```python
from build123d import *

# Parameters (mm, degrees)
F0_W          = 30
F0_H          = 50
F1_DEPTH      = 10
F2_R          = 10.0991386475
F3_DEPTH      = 10
F4_R          = 4.0969126616
F5_DEPTH      = 25
F5_DEPTH_BACK = 25
F6_SIZE       = 0.5
F7_SIZE       = 0.5


# Not quite as in the source:
# - a feature names something its author has since deleted; it is built from what else it names


with BuildPart() as f1:
    # F0 (on Top) → F1 (new body)
    with BuildSketch(Plane.XY):
        Rectangle(F0_W, F0_H)
    extrude(amount=-F1_DEPTH)

    # F2 (on Top) → F3 (join)
    with BuildSketch(Plane.XY):
        Circle(F2_R)
    extrude(amount=F3_DEPTH)

    # F4 (on Top) → F5 (cut, two sides)
    with BuildSketch(Plane.XY) as f5_sk:
        Circle(F4_R)
    extrude(amount=-F5_DEPTH, mode=Mode.SUBTRACT)
    extrude(f5_sk.sketch, amount=F5_DEPTH_BACK, mode=Mode.SUBTRACT)

    # F6
    f6_edges = [f1.edges().sort_by_distance(p)[0] for p in [
        (15, 0, 0),
        (0, -25, 0),
        (-15, 0, 0),
        (0, 25, 0),
        (-10.099139, 0, 10),
        (-4.096913, 0, 10),
        (15, -25, -5),
        (15, 25, -5),
        (-15, -25, -5),
        (0, -25, -10),
        (15, 0, -10),
        (-15, 25, -5),
        (-15, 0, -10),
        (0, 25, -10),
    ]]
    chamfer(f6_edges, length=F6_SIZE)

    # F7
    f7_edges = [f1.edges().sort_by_distance(p)[0] for p in [
        (-4.096913, 0, -10),
    ]]
    chamfer(f7_edges, length=F7_SIZE)


solid = f1.part
```
The listing builds one solid part. Answer for the finished solid, in the listing's coordinates (mm). Give positions to 0.01 mm unless a question says otherwise; leave off trailing zeros. Order: outer loops, then holes, each group sorted by start corner. A loop starts at its lowest first (then second) coordinate and runs counter-clockwise, first axis right, second up.
Item 1: Find the intervals of material crossed by probe 1 along Y at (x, z) = (0, 0.5); probe 2 along X at (y, z) = (0, -3.5); probe 3 along Z at (x, y) = (-13, 23.5), in increasing order.
From the geometry:
probe 1: y = -10.1 to -4.1, 4.1 to 10.1
probe 2: x = -15 to -4.1, 4.1 to 15
probe 3: z = -10 to 0
Item 2: Given pin 1 Ø6 at (y, z) = (11, 7.5) entering from +X; pin 2 Ø1 at (x, y) = (0, -4) entering from -Z; pin 3 Ø5 at (x, y) = (-10, 12) entering from +Z; pin 4 Ø5 at (x, y) = (0, 0) entering from +Z, each flat-ended and moving along its own axis, determine where each tip first touches the part or whether it passes through.
From the geometry:
pin 1: stops at x = 6.16
pin 2: stops at z = -9.9
pin 3: stops at z = 0
pin 4: passes through
Item 3: For a pull along Y with two mould halves and no side action, classify faces 1 (the face through (0, 6, -10)), 2 (the face through (0, 25, -5)), 3 (the face through (9.633, 3.034, 4.684)), 4 (the face through (3.91, 1.23, 0.13)) as pulls with the +Y half, pulls with the -Y half, needs draft (parallel to the pull), parting line crosses it, or undercut.
From the geometry:
face 1: needs draft
face 2: pulls with the +Y half
face 3: parting line crosses it
face 4: undercut
Item 4: The part is cut by section D-D, the plane y = 14. Give the vertices of the cut face in (x, z).
From the geometry:
outline: (-15, -9.5) - (-14.5, -10) - (14.5, -10) - (15, -9.5) - (15, -0.5) - (14.5, 0) - (-14.5, 0) - (-15, -0.5) - close
Item 5: The part is cut by section C-C, the plane z = -5.25. Give the vertices of the cut face in (x, y), and give its area (3 significant figures).
From the geometry:
outline: (-15, -24.5) - (-14.5, -25) - (14.5, -25) - (15, -24.5) - (15, 24.5) - (14.5, 25) - (-14.5, 25) - (-15, 24.5) - close; hole circle Ø8.19 at (0, 0)
area: 1,450 mm2
Item 6: The part is cut by section B-B, the plane x = 0. Give the vertices of the cut face in (y, z).
From the geometry:
outline: (-25, -9.5) - (-24.5, -10) - (-4.6, -10) - (-4.1, -9.5) - (-4.1, 9.5) - (-4.6, 10) - (-9.6, 10) - (-10.1, 9.5) - (-10.1, 0) - (-24.5, 0) - (-25, -0.5) - close; (4.1, -9.5) - (4.6, -10) - (24.5, -10) - (25, -9.5) - (25, -0.5) - (24.5, 0) - (10.1, 0) - (10.1, 9.5) - (9.6, 10) - (4.6, 10) - (4.1, 9.5) - close
Item 7: The part is cut by section A-A, the plane y = 0. Give the vertices of the cut face in (x, z).
From the geometry:
outline: (-15, -9.5) - (-14.5, -10) - (-4.6, -10) - (-4.1, -9.5) - (-4.1, 9.5) - (-4.6, 10) - (-9.6, 10) - (-10.1, 9.5) - (-10.1, 0) - (-14.5, 0) - (-15, -0.5) - close; (4.1, -9.5) - (4.6, -10) - (14.5, -10) - (15, -9.5) - (15, -0.5) - (14.5, 0) - (10.1, 0) - (10.1, 9.5) - (9.6, 10) - (4.6, 10) - (4.1, 9.5) - close
